```python
from build123d import *

# Parameters (mm, degrees)
BOSS_EXTRUDE1_DEPTH = 31.5
SHELL1_T            = -1
BOSS_EXTRUDE2_DEPTH = 30.5
BOSS_EXTRUDE4_START = -6.3
BOSS_EXTRUDE4_DEPTH = 6.3
SKETCH5_R           = 1.5
CUT_EXTRUDE2_DEPTH  = 5


with BuildPart() as part:
    # Sketch1 → Boss-Extrude1 (new body)
    with BuildSketch(Plane(origin=(0, 0, 0), x_dir=(1, 0, 0), z_dir=(0, 1, 0))):
        with BuildLine():
            Line((-68.5, -21.25), (-68.5, 21.25))
            ThreePointArc((-68.5, 21.25), (-67.621320344, 23.371320344), (-65.5, 24.25))
            Line((-65.5, 24.25), (65.5, 24.25))
            ThreePointArc((65.5, 24.25), (67.621320344, 23.371320344), (68.5, 21.25))
            Line((68.5, 21.25), (68.5, -21.25))
            ThreePointArc((68.5, -21.25), (67.621320344, -23.371320344), (65.5, -24.25))
            Line((65.5, -24.25), (-65.5, -24.25))
            ThreePointArc((-65.5, -24.25), (-67.621320344, -23.371320344), (-68.5, -21.25))
        make_face()
    extrude(amount=BOSS_EXTRUDE1_DEPTH)

    # Shell1
    shell1_openings = [part.faces().sort_by_distance(p)[0] for p in [
        (0, 0, 0),
    ]]
    offset(amount=SHELL1_T, openings=shell1_openings, kind=Kind.INTERSECTION)

    # Sketch2 → Boss-Extrude2 (add)
    with BuildSketch(Plane(origin=(0, 0, 0), x_dir=(1, 0, 0), z_dir=(0, 1, 0))):
        with BuildLine():
            Line((-68.5, 21.25), (-68.5, 17))
            Line((-68.5, 17), (-63.5, 17))
            ThreePointArc((-63.5, 17), (-61.909009742, 17.659009742), (-61.25, 19.25))
            Line((-61.25, 19.25), (-61.25, 24.25))
            Line((-61.25, 24.25), (-65.5, 24.25))
            ThreePointArc((-65.5, 24.25), (-67.621320344, 23.371320344), (-68.5, 21.25))
        make_face()
        with BuildLine():
            Line((-65.5, -24.25), (-61.25, -24.25))
            Line((-61.25, -24.25), (-61.25, -19.25))
            ThreePointArc((-61.25, -19.25), (-61.909009742, -17.659009742), (-63.5, -17))
            Line((-63.5, -17), (-68.5, -17))
            Line((-68.5, -17), (-68.5, -21.25))
            ThreePointArc((-68.5, -21.25), (-67.621320344, -23.371320344), (-65.5, -24.25))
        make_face()
        with BuildLine():
            Line((68.5, 21.25), (68.5, 17))
            Line((68.5, 17), (63.5, 17))
            ThreePointArc((63.5, 17), (61.909009742, 17.659009742), (61.25, 19.25))
            Line((61.25, 19.25), (61.25, 24.25))
            Line((61.25, 24.25), (65.5, 24.25))
            ThreePointArc((65.5, 24.25), (67.621320344, 23.371320344), (68.5, 21.25))
        make_face()
        with BuildLine():
            Line((61.25, -19.25), (61.25, -24.25))
            Line((61.25, -24.25), (65.5, -24.25))
            ThreePointArc((65.5, -24.25), (67.621320344, -23.371320344), (68.5, -21.25))
            Line((68.5, -21.25), (68.5, -17))
            Line((68.5, -17), (63.5, -17))
            ThreePointArc((63.5, -17), (61.909009742, -17.659009742), (61.25, -19.25))
        make_face()
    extrude(amount=BOSS_EXTRUDE2_DEPTH)

    # Sketch4 → Boss-Extrude4 (add)
    with BuildSketch(Plane(origin=(0, 0, 0), x_dir=(1, 0, 0), z_dir=(0, 1, 0)).offset(BOSS_EXTRUDE4_START)):
        with BuildLine():
            Line((-68.5, -21.25), (-68.5, 21.25))
            ThreePointArc((-68.5, 21.25), (-67.621320344, 23.371320344), (-65.5, 24.25))
            Line((-65.5, 24.25), (65.5, 24.25))
            ThreePointArc((65.5, 24.25), (67.621320344, 23.371320344), (68.5, 21.25))
            Line((68.5, 21.25), (68.5, -21.25))
            ThreePointArc((68.5, -21.25), (67.621320344, -23.371320344), (65.5, -24.25))
            Line((65.5, -24.25), (-65.5, -24.25))
            ThreePointArc((-65.5, -24.25), (-67.621320344, -23.371320344), (-68.5, -21.25))
        make_face()
        with BuildLine():
            Line((-65.5, -23.25), (65.5, -23.25))
            ThreePointArc((65.5, -23.25), (66.914213562, -22.664213562), (67.5, -21.25))
            Line((67.5, -21.25), (67.5, 21.25))
            ThreePointArc((67.5, 21.25), (66.914213562, 22.664213562), (65.5, 23.25))
            Line((65.5, 23.25), (-65.5, 23.25))
            ThreePointArc((-65.5, 23.25), (-66.914213562, 22.664213562), (-67.5, 21.25))
            Line((-67.5, 21.25), (-67.5, -21.25))
            ThreePointArc((-67.5, -21.25), (-66.914213562, -22.664213562), (-65.5, -23.25))
        make_face(mode=Mode.SUBTRACT)
    extrude(amount=BOSS_EXTRUDE4_DEPTH)

    # Sketch5 → Cut-Extrude2 (cut)
    with BuildSketch(Plane.XZ):
        with Locations(Location((-63.5, 19.25, 0), (0, 0, 270))):
            Circle(SKETCH5_R)
        with Locations(Location((-63.5, -19.25, 0), (0, 0, 270))):
            Circle(SKETCH5_R)
        with Locations(Location((63.5, 19.25, 0), (0, 0, 270))):
            Circle(SKETCH5_R)
        with Locations(Location((63.5, -19.25, 0), (0, 0, 270))):
            Circle(SKETCH5_R)
    extrude(amount=-CUT_EXTRUDE2_DEPTH, mode=Mode.SUBTRACT)


solid = part.part
```
Can you work these out from the model? Positions are in its coordinate system, mm. A direction names the side the tool comes from. Coordinates: 2 decimals unless noted, no trailing zeros. Loops run counter-clockwise (first coordinate to the right, second up) from the corner with the lowest first, then second, coordinate; pieces in that order, holes last. Notation, with made-up numbers: (-17, 16) -> (8, 16) arc R4 ccw to (8, 21) -> close; hole circle Ø6 at (-4, 67.25). An arc over 180 degrees is marked (long way). Answer as a JSON object with one key per item and string values.
1) For P1, Ø1.8, axis at x = -63.5, z = -19.25, coming from the -Y side; P2, Ø6, axis at x = 44, z = 1, coming from the -Y side; P3, Ø2.5, axis at x = -64, z = 19, coming from the -Y side, each with a flat end and sliding along its axis, tell me the tip position at first contact or that it passes through.
Results:
{"P1": "stops at y = 5", "P2": "stops at y = 30.5", "P3": "stops at y = 0"}
2) Thinking about a two-plate mould opening in Z: for faces 3 (the face through (-1, 12, 23.25)), 4 (the face through (1, 31.5, 0)), 5 (the face through (1, 12, 24.25)), which applies, pulls with the +Z half, pulls with the -Z half, needs draft (parallel to the pull), parting line crosses it, or undercut?
Results:
{"face 3": "undercut", "face 4": "needs draft", "face 5": "pulls with the +Z half"}
3) If I drill on line 1 (X direction, y = 1.6, z = -19.25); line 2 (Z direction, x = -44.5, y = 2.5), over which ranges is the centre line in solid material (lowest first)?
Results:
{"line 1": "x = -68.5 to -65, -62 to -61.25, 61.25 to 62, 65 to 68.5", "line 2": "z = -24.25 to -23.25, 23.25 to 24.25"}
4) Imagine slicing it at C-C (x = 1). Please give me the cut outline in (y, z), then the cut area to 3 significant figures.
Results:
{"outline": "(-6.3, -24.25) -> (31.5, -24.25) -> (31.5, 24.25) -> (-6.3, 24.25) -> (-6.3, 23.25) -> (30.5, 23.25) -> (30.5, -23.25) -> (-6.3, -23.25) -> close", "area": "122 mm^2"}
5) For faces 1 (the face through (61.25, 15, 21)), 2 (the face through (-1, 12, -24.25)), which set-ups out of +Z, -Z, +X, -X, +Y, -Y let a thin tool reach every point of the face, with its end or its side?
Results:
{"face 1": "-Y", "face 2": "-Z, +X, -X, +Y, -Y"}
6) Imagine slicing it at B-B (z = -14). Please give me the cut outline in (x, y).
Results:
{"outline": "(-68.5, -6.3) -> (-67.5, -6.3) -> (-67.5, 30.5) -> (67.5, 30.5) -> (67.5, -6.3) -> (68.5, -6.3) -> (68.5, 31.5) -> (-68.5, 31.5) -> close"}
7) Imagine slicing it at A-A (y = 11.5). Please give me the cut outline in (x, z), then the cut area to 3 significant figures.
Results:
{"outline": "(-68.5, -21.25) arc R3 ccw to (-65.5, -24.25) -> (65.5, -24.25) arc R3 ccw to (68.5, -21.25) -> (68.5, 21.25) arc R3 ccw to (65.5, 24.25) -> (-65.5, 24.25) arc R3 ccw to (-68.5, 21.25) -> close; hole (-67.5, -17) -> (-63.5, -17) arc R2.25 cw to (-61.25, -19.25) -> (-61.25, -23.25) -> (61.25, -23.25) -> (61.25, -19.25) arc R2.25 cw to (63.5, -17) -> (67.5, -17) -> (67.5, 17) -> (63.5, 17) arc R2.25 cw to (61.25, 19.25) -> (61.25, 23.25) -> (-61.25, 23.25) -> (-61.25, 19.25) arc R2.25 cw to (-63.5, 17) -> (-67.5, 17) -> close", "area": "511 mm^2"}
